Here's how the part is built. I have some questions about the finished solid (model axes, mm). A direction names the side the tool comes from. Coordinates: 2 decimals unless noted, no trailing zeros. Write each loop counter-clockwise with the first axis right and the second up, starting at its lowest first coordinate (ties: lowest second). Pieces come first, ordered by that corner, then holes. Notation, with made-up numbers: M -37.75,40 L 8.25,40 A22 cw 8.25,71 Z; hole C 35,-17 d1. An arc over 180 degrees is marked long. Use one line per item in the form item = value. Start each with the question number.
1. Thinking about a two-plate mould opening in Z: for faces 1 (the face through (14.13, 21.4, 1.38)), 2 (the face through (11.5, 0, -2)), 3 (the face through (0, 0, -4)), which applies, released by +Z, released by -Z, zero draft, split by the parting line, or undercut?
2. I want a section at C-C, the plane y = -21.5. List the corners of the cut face in (x, z) for me, plus the area to 3 significant figures.
3. On a 3-axis mill with a long thin cutter (end or side, diameter ignored), from which of +Z, -Z, +X, -X, +Y, -Y can I reach the whole of each face in a straight line? I mean faces 4 (the face through (21, 14, 0)), 5 (the face through (0, 0, 0)), 6 (the face through (14.13, -21.6, 1.38)). Say none if no direction works.
4. I'm going to push flat-ended pins straight in: pin 1 Ø11.5 at (x, y) = (0, -8) entering from +Z; pin 2 Ø5 at (x, z) = (-6, 4) entering from -Y; pin 3 Ø1.2 at (y, z) = (2, -2.5) entering from +X; pin 4 Ø6 at (y, z) = (22.5, 8) entering from -X. Where does each tip first touch, or does it pass through?
5. Please list where these lines run through material, in increasing order: line 1 along Y through (x, z) = (-9.5, -2.2); line 2 along Y through (x, z) = (12, 4.5); line 3 along X through (y, z) = (17.5, 4). Write a range as [from, to].
6. I want a section at D-D, the plane z = -2. List the corners of the cut face in (x, y) for me.
7. I want a section at A-A, the plane z = 4. List the corners of the cut face in (x, y) for me, plus the area to 3 significant figures.
8. I want a section at B-B, the plane x = 20.5. List the corners of the cut face in (y, z) for me.
from build123d import *

# Parameters (mm, degrees)
BASE_FLANGE1_DEPTH = 4
HEM2_START         = -29
HEM2_DEPTH         = 15
HEM2_START_2       = 14
HEM2_2_DEPTH       = 15
SKETCH16_R         = 4.5
CUT_EXTRUDE1_DEPTH = 10
FILLET1_R          = 10


# Read off the part's stored shape, not the designer's step: Hem2
# Sheet-metal steps are written as plain solids
with BuildPart() as part:
    # Sketch1 → Base-Flange1 (new body)
    with BuildSketch(Plane.XY):
        Polygon((-19.5, 29), (19.5, 29), (19.5, 14), (11.5, 14), (11.5, -14), (19.5, -14), (19.5, -29), (-19.5, -29), align=None)
    extrude(amount=-BASE_FLANGE1_DEPTH)

    # Hem2 outline → Hem2 (add)
    with BuildSketch(Plane(origin=(0, 0, 0), x_dir=(1, 0, 0), z_dir=(0, 1, 0)).offset(HEM2_START)):
        with BuildLine():
            Line((15.904823815, -2.246515413), (12.30964763, -0.493030826))
            ThreePointArc((12.30964763, -0.493030826), (23.739354115, -10.784384769), (19.5, 4))
            Line((19.5, 4), (19.5, 0))
            ThreePointArc((19.5, 0), (21.619677058, -7.392192385), (15.904823815, -2.246515413))
        make_face()
    extrude(amount=HEM2_DEPTH)

    # Hem2 2 outline → Hem2 2 (add)
    with BuildSketch(Plane(origin=(0, 0, 0), x_dir=(1, 0, 0), z_dir=(0, 1, 0)).offset(HEM2_START_2)):
        with BuildLine():
            Line((15.904823815, -2.246515413), (12.30964763, -0.493030826))
            ThreePointArc((12.30964763, -0.493030826), (23.739354115, -10.784384769), (19.5, 4))
            Line((19.5, 4), (19.5, 0))
            ThreePointArc((19.5, 0), (21.619677058, -7.392192385), (15.904823815, -2.246515413))
        make_face()
    extrude(amount=HEM2_2_DEPTH)

    # Sketch16 → Cut-Extrude1 (cut)
    with BuildSketch(Plane.XY):
        with Locations((-9.5, 18.5)):
            Circle(SKETCH16_R)
        with Locations((-9.5, -18.5)):
            Circle(SKETCH16_R)
    extrude(amount=-CUT_EXTRUDE1_DEPTH, mode=Mode.SUBTRACT)

    # Fillet1
    fillet1_edges = [part.edges().sort_by_distance(p)[0] for p in [
        (-19.5, -29, -2),
        (-19.5, 29, -2),
    ]]
    fillet(fillet1_edges, radius=FILLET1_R)


solid = part.part
Answer list:
q1.face_1 = undercut
q1.face_2 = zero draft
q1.face_3 = released by -Z
q2.outline = M -19.18,-4 L -12.85,-4 L -12.85,0 L -19.18,0 Z; M -6.15,-4 L 19.5,-4 A8 ccw long 12.31,0.49 L 15.9,2.25 A4 cw long 19.5,0 L -6.15,0 Z
q2.area = 252 mm²
q3.face_4 = +Z, -Z, +X
q3.face_5 = -X, +Y, -Y
q3.face_6 = +Y, -Y
q4.pin_1 = 0
q4.pin_2 = through
q4.pin_3 = 11.5
q4.pin_4 = 11.56
q5.line_1 = [-29, -23], [-14, 14], [23, 29]
q5.line_2 = [-29, -14], [14, 29]
q5.line_3 = [11.5, 15.5], [23.5, 27.5]
q6.outline = M -19.5,-19 A10 ccw -9.5,-29 L 24.79,-29 L 24.79,-14 L 11.5,-14 L 11.5,14 L 24.79,14 L 24.79,29 L -9.5,29 A10 ccw -19.5,19 Z; hole C -9.5,-18.5 d9; hole C -9.5,18.5 d9
q7.outline = M 11.5,-29 L 15.5,-29 L 15.5,-14 L 11.5,-14 Z; M 11.5,14 L 15.5,14 L 15.5,29 L 11.5,29 Z; M 23.5,-29 L 27.5,-29 L 27.5,-14 L 23.5,-14 Z; M 23.5,14 L 27.5,14 L 27.5,29 L 23.5,29 Z
q7.area = 240 mm²
q8.outline = M -29,-3.94 L -14,-3.94 L -14,0.13 L -29,0.13 Z; M -29,7.87 L -14,7.87 L -14,11.94 L -29,11.94 Z; M 14,-3.94 L 29,-3.94 L 29,0.13 L 14,0.13 Z; M 14,7.87 L 29,7.87 L 29,11.94 L 14,11.94 Z
